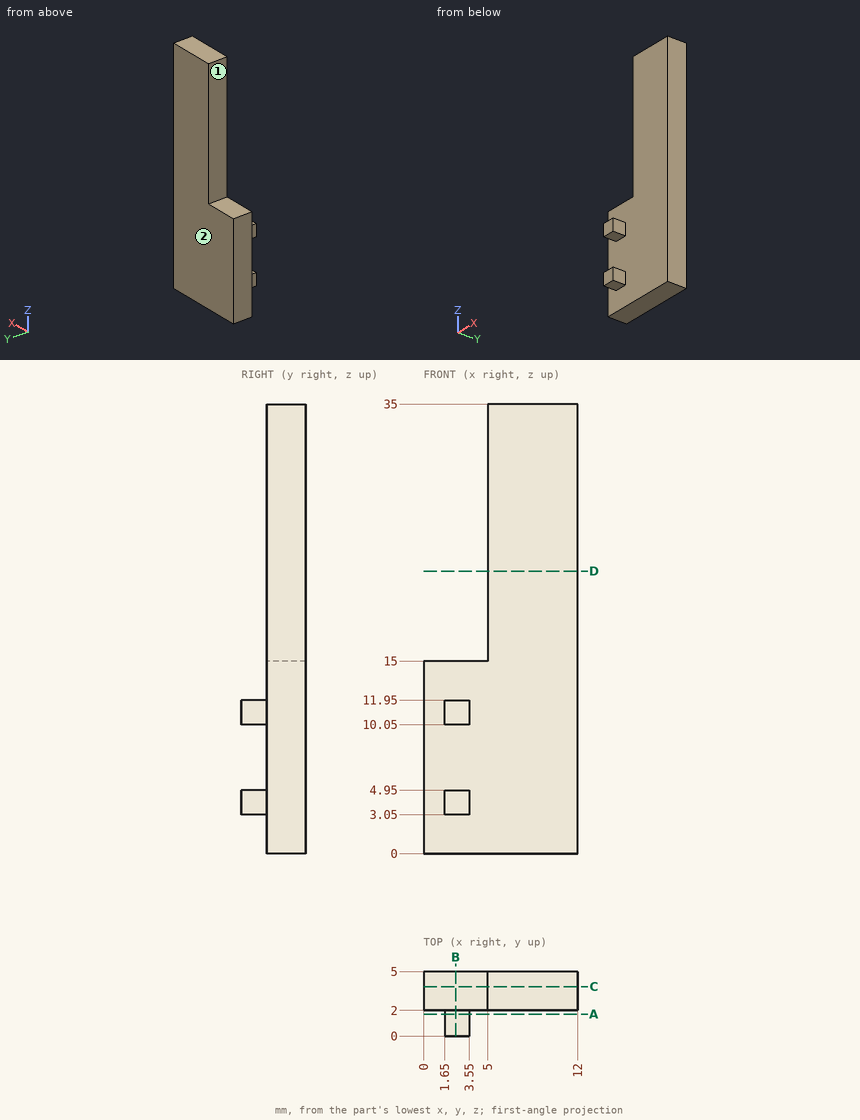
Could you check a few things on this drawing? It's one solid part, dimensions in mm from its lowest x, y, z. A direction names the side the tool comes from. Round coordinates to 2 decimals unless told otherwise and drop trailing zeros. Order: outer loops, then holes, each group sorted by start corner. A loop starts at its lowest first (then second) coordinate and runs counter-clockwise, first axis right, second up. Notation, with made-up numbers: M 72.25,20.5 L 104.25,20.5 A15 ccw 104.25,30.5 Z; hole C 41,53 d1. An arc over 180 degrees is marked long. Return JSON: item names as keys, results as strings. Group by question number.
1. Please list where these lines run through material, in increasing order: probe 1 along Z at (x, y) = (3, 1.7); probe 2 along X at (y, z) = (2.5, 33.5); probe 3 along Y at (x, z) = (3.75, 2).
2. I'm going to push flat-ended pins straight in: pin 1 Ø1.5 at (x, y) = (2.5, 1) entering from +Z; pin 2 Ø1.5 at (y, z) = (0.5, 4) entering from +X; pin 3 Ø3 at (y, z) = (3, 18) entering from -X; pin 4 Ø6 at (x, z) = (4, 24) entering from +Y. Where does each tip first touch, or does it pass through?
3. If we section it at D-D on z = 22: List the corners of the cut face in (x, y) for me.
4. If we section it at B-B on x = 2.5: List the corners of the cut face in (y, z) for me.
5. On a 3-axis mill with a long thin cutter (end or side, diameter ignored), from which of +Z, -Z, +X, -X, +Y, -Y can I reach the whole of each face in a straight line? I mean the marked faces 1 and 2. Say none if no direction works.
6. If we section it at C-C on y = 3.85: List the corners of the cut face in (x, z) for me.
7. If we section it at A-A on y = 1.7: List the corners of the cut face in (x, z) for me.
Reply:
{
 "1": {"probe 1": "3.05 to 4.95, 10.05 to 11.95", "probe 2": "5 to 12", "probe 3": "2 to 5"},
 "2": {"pin 1": "z = 11.95", "pin 2": "x = 3.55", "pin 3": "x = 5", "pin 4": "y = 5"},
 "3": {"outline": "M 5,2 L 12,2 L 12,5 L 5,5 Z"},
 "4": {"outline": "M 0,3.05 L 2,3.05 L 2,0 L 5,0 L 5,15 L 2,15 L 2,11.95 L 0,11.95 L 0,10.05 L 2,10.05 L 2,4.95 L 0,4.95 Z"},
 "5": {"face 1": "+Z, -X, +Y, -Y", "face 2": "+Z, -Z, +X, -X, +Y"},
 "6": {"outline": "M 0,0 L 12,0 L 12,35 L 5,35 L 5,15 L 0,15 Z"},
 "7": {"outline": "M 1.65,3.05 L 3.55,3.05 L 3.55,4.95 L 1.65,4.95 Z; M 1.65,10.05 L 3.55,10.05 L 3.55,11.95 L 1.65,11.95 Z"}
}
